Work out the finished part from the listing and answer in its coordinate system (mm). Face numbers are marked on the shaded views. A direction names the side the tool comes from. Round coordinates to 2 decimals unless told otherwise and drop trailing zeros. Order: outer loops, then holes, each group sorted by start corner. A loop starts at its lowest first (then second) coordinate and runs counter-clockwise, first axis right, second up. Notation, with made-up numbers: (14, -15) - (66, -15) arc R28 cw to (66, 12) - close; hole circle Ø11 at (50.25, 61). An arc over 180 degrees is marked (long way). Put each result on its own line as item: value.
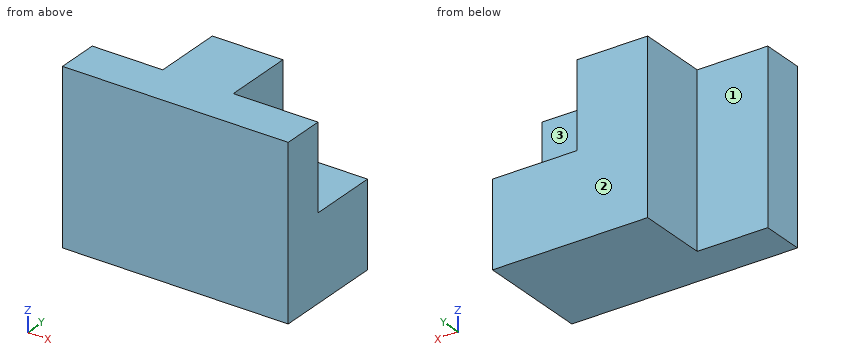
```python
from build123d import *

# Parameters (mm, degrees)
F0_W     = 80
F0_H     = 60
F1_DEPTH = 15
F3_DEPTH = 25


with BuildPart() as f1:
    # F0 (on Front) → F1 (new body)
    with BuildSketch(Plane.XZ):
        with Locations((-40, 30)):
            Rectangle(F0_W, F0_H)
    extrude(amount=F1_DEPTH)

    # F2 (on Front) → F3 (join)
    with BuildSketch(Plane.XZ):
        Polygon((-55, 0), (0, 0), (0, 30), (-30, 30), (-30, 60), (-55, 60), (-55, 53.417352), align=None)
    extrude(amount=-F3_DEPTH)


solid = f1.part
```
1) Straight lines are drawn through the part: L1, parallel to Y at x = -7, z = 49.5; L2, parallel to X at y = 2.5, z = 30.5; L3, parallel to X at y = 18.5, z = 21. For each, find the intervals that lie inside material, in ascending order. Write a range as from..to.
Findings below:
L1: y = -15..0
L2: x = -55..-30
L3: x = -55..0
2) Given pin 1 Ø7.5 at (y, z) = (12.5, 45) entering from +X; pin 2 Ø5 at (y, z) = (8, 11.5) entering from -X; pin 3 Ø4 at (x, z) = (-13, 33) entering from +Y, each flat-ended and moving along its own axis, determine where each tip first touches the part or whether it passes through.
Findings below:
pin 1: stops at x = -30
pin 2: stops at x = -55
pin 3: stops at y = 0
3) A cutting plane is placed at A-A on z = 46.5. Write down the section's boundary in (x, y), then the cut area to 4 significant figures.
Findings below:
outline: (-80, -15) - (0, -15) - (0, 0) - (-30, 0) - (-30, 25) - (-55, 25) - (-55, 0) - (-80, 0) - close
area: 1,825 mm2
4) A cutting plane is placed at B-B on x = -16.5. Write down the section's boundary in (y, z), then the cut area to 3 significant figures.
Findings below:
outline: (-15, 0) - (25, 0) - (25, 30) - (0, 30) - (0, 60) - (-15, 60) - close
area: 1,650 mm2
5) For the marked faces 1, 2 and 3, determine the directions among +Z, -Z, +X, -X, +Y, -Y from which every point of the face is accessible in a straight line to the end or side of a thin tool.
Findings below:
face 1: +Z, -Z, -X, +Y
face 2: +Z, -Z, +X, -X, +Y
face 3: +Z, +X, +Y
6) A cutting plane is placed at D-D on x = -62.5. Write down the section's boundary in (y, z).
Findings below:
outline: (-15, 0) - (0, 0) - (0, 60) - (-15, 60) - close
7) A cutting plane is placed at C-C on z = 26.5. Write down the section's boundary in (x, y), then the cut area to 4 significant figures.
Findings below:
outline: (-80, -15) - (0, -15) - (0, 25) - (-55, 25) - (-55, 0) - (-80, 0) - close
area: 2,575 mm2
